Source: CAD feature listing. Evaluate the final solid. Frame: model axes, mm. Give positions to 0.01 mm unless a question says otherwise; leave off trailing zeros. Order: outer loops, then holes, each group sorted by start corner. A loop starts at its lowest first (then second) coordinate and runs counter-clockwise, first axis right, second up. Notation, with made-up numbers: M 40.25,12.25 L 63.25,12.25 A19 ccw 63.25,24.25 Z; hole C 71.5,62.5 d2. An arc over 180 degrees is marked long. Use CSV: the item, a comma, the result in double quotes. Start each with the question number.
1. Line query: line 1 along Y through (x, z) = (-10, 2); line 2 along X through (y, z) = (10.5, 0.85); line 3 along X through (y, z) = (11.3, 2.1). Output: solid intervals per line, ascending. Write a range as [from, to].
2. Section query B-B, the plane z = 0.9. Return the cut outline in (x, y).
3. Section query C-C, the plane y = 11.3. Return the cut outline in (x, z), plus the area to 3 significant figures.
4. Mould query, pull axis Y, two halves, no side actions, for faces 1 (the flat face through (22.9, -4, 1)), 2 (the cylindrical face through (6.7, 11.2, 1.5)), 3 (the flat face through (19.36, 13.44, 1.48)), 4 (the cylindrical face through (-22.187, -17.748, 1.521)). Classes: released by +Y, released by -Y, zero draft, split by the parting line, or undercut.
5. Section query D-D, the plane x = 19.5. Return the cut outline in (y, z).
6. Pin query (flat end, axial travel): P1, Ø5.5, axis at x = 10, y = 11.3, coming from the +Z side. Return the tip coordinate at first contact, or that it passes through.
7. Section query A-A, the plane x = 10. Return the cut outline in (y, z), plus the area to 3 significant figures.
Autodesk Fusion 360 part; units mm, degrees
sketch "Sketch1" plane through (0, 0, 0) normal (0, 0, 1) x (1, 0, 0)
  line L0 (22.9, -18.5) -> (-22.9, -18.5)
  line L1 (-22.9, -18.5) -> (-22.9, 8.8)
  line L2 (-15.5, 18.5) -> (15.5, 18.5)
  line L3 (22.9, 8.8) -> (22.9, -18.5)
  line L4 (22.9, -18.5) -> (-22.9, 18.5) construction
  line L5 (-22.9, -18.5) -> (22.9, 18.5) construction
  line L6 (0, 18.5) -> (0, -18.5)
  line L7 (10, 14.6) -> (10, 8)
  circle A0 centre (-10, 11.3) radius 3.3
  circle A1 centre (10, 11.3) radius 3.3
  line L8 (-22.9, 8.8) -> (-15.5, 18.5)
  line L9 (22.9, 8.8) -> (15.5, 18.5)
  line L10 (-13.9876, 11.3) -> (-13.3, 11.3)
  line L11 (13.3, 11.3) -> (13.9876, 11.3)
  line L12 (-10, 8.0786) -> (-10, 8)
  dimension "d1" = 45.8
  dimension "d2" = 37
  dimension "d5" = 6.6
  dimension "d6" = 27.3
extrude "Extrude1" add sketch "Sketch1" along normal blind 3
fillet "Fillet1" radius 2.5 6 edges at (15.5, 18.5, 1.5) (22.9, 8.8, 1.5) (22.9, -18.5, 1.5) (-22.9, -18.5, 1.5) (-22.9, 8.8, 1.5) (-15.5, 18.5, 1.5)
Result set:
1,line 1,"[-18.5, 8], [14.6, 18.5]"
1,line 2,"[-21.6, -13.2], [-6.8, 6.8], [13.2, 21.6]"
1,line 3,"[-20.99, -13.3], [-6.7, 6.7], [13.3, 20.99]"
2,outline,"M -22.9,-16 A2.5 ccw -20.4,-18.5 L 20.4,-18.5 A2.5 ccw 22.9,-16 L 22.9,7.96 A2.5 ccw 22.39,9.47 L 16.25,17.52 A2.5 ccw 14.26,18.5 L -14.26,18.5 A2.5 ccw -16.25,17.52 L -22.39,9.47 A2.5 ccw -22.9,7.96 Z; hole C -10,11.3 d6.6; hole C 10,11.3 d6.6"
3,outline,"M -20.99,0 L -13.3,0 L -13.3,3 L -20.99,3 Z; M -6.7,0 L 6.7,0 L 6.7,3 L -6.7,3 Z; M 13.3,0 L 20.99,0 L 20.99,3 L 13.3,3 Z"
3,area,"86.4 mm2"
4,face 1,"zero draft"
4,face 2,"undercut"
4,face 3,"released by +Y"
4,face 4,"released by -Y"
5,outline,"M -18.5,0 L 13.26,0 L 13.26,3 L -18.5,3 Z"
6,P1,"through"
7,outline,"M -18.5,0 L 8,0 L 8,3 L -18.5,3 Z; M 14.6,0 L 18.5,0 L 18.5,3 L 14.6,3 Z"
7,area,"91.2 mm2"
